Here's how the part is built. I have some questions about the finished solid (model axes, mm). Face numbers are marked on the shaded views. Round coordinates to 2 decimals unless told otherwise and drop trailing zeros. Write each loop counter-clockwise with the first axis right and the second up, starting at its lowest first coordinate (ties: lowest second). Pieces come first, ordered by that corner, then holes. Notation, with made-up numbers: (67.5, -27) -> (87.5, -27) arc R27 ccw to (87.5, 0) -> close; hole circle Ø6 at (73.25, 22). An arc over 180 degrees is marked (long way). Put each result on its own line as item: value. Start each with the question number.
1) If I drill on line 1 along Z through (x, y) = (-20, 6.5); line 2 along Z through (x, y) = (34, -0.5); line 3 along X through (y, z) = (5, -7.25), over which ranges is the centre line in solid material (lowest first)? Write a range as [from, to].
2) I want a section at C-C, the plane z = -9. List the corners of the cut face in (x, y) for me, then the cut area to 3 significant figures.
3) I want a section at A-A, the plane x = -5. List the corners of the cut face in (y, z) for me.
4) I want a section at B-B, the plane y = 5. List the corners of the cut face in (x, z) for me, then the cut area to 3 significant figures.
5) Will these pins go through, and if not, where does the flat tip stop? P1, Ø0.6, axis at y = 9, z = 1.5, coming from the +X side; P2, Ø8, axis at x = -8, z = -2, coming from the +Y side; P3, Ø4, axis at x = 14.5, y = 5, coming from the +Z side; P4, Ø1.6, axis at x = -33, z = 1.5, coming from the -Y side.
6) We'd pull the mould along Z, two halves only. Please class the marked faces 1 and 2: released by +Z, released by -Z, zero draft, split by the parting line, or undercut.
from build123d import *

# Parameters (mm, degrees)
SKIZZE1_W                            = 155
SKIZZE1_H                            = 23
SKIZZE1_W_2                          = 147
SKIZZE1_H_2                          = 15
AUFSATZ_LINEAR_AUSTRAGEN1_DEPTH      = 10
SKIZZE2_W                            = 2
SKIZZE2_H                            = 15
AUFSATZ_LINEAR_AUSTRAGEN2_DEPTH      = 2
AUFSATZ_LINEAR_AUSTRAGEN3_DEPTH      = 1.5
AUFSATZ_LINEAR_AUSTRAGEN3_DEPTH_BACK = 2
SKIZZE3_W                            = 159
SKIZZE3_H                            = 27
SKIZZE3_W_2                          = 155
SKIZZE3_H_2                          = 23


with BuildPart() as part:
    # Skizze1 → Aufsatz-Linear austragen1 (new body)
    with BuildSketch(Plane(origin=(0, 0, 0), x_dir=(1, 0, 0), z_dir=(0, 1, 0))):
        Rectangle(SKIZZE1_W, SKIZZE1_H)
        Rectangle(SKIZZE1_W_2, SKIZZE1_H_2, mode=Mode.SUBTRACT)
    extrude(amount=AUFSATZ_LINEAR_AUSTRAGEN1_DEPTH)

    # Skizze2 → Aufsatz-Linear austragen2 (add)
    with BuildSketch(Plane(origin=(0, 10, 0), x_dir=(1, 0, 0), z_dir=(0, 1, 0))):
        with Locations((-52.5, 0)):
            Rectangle(SKIZZE2_W, SKIZZE2_H)
        with Locations((-32.5, 0)):
            Rectangle(SKIZZE2_W, SKIZZE2_H)
        with Locations((-12.5, 0)):
            Rectangle(SKIZZE2_W, SKIZZE2_H)
        with Locations((7.5, 0)):
            Rectangle(SKIZZE2_W, SKIZZE2_H)
        with Locations((27.5, 0)):
            Rectangle(SKIZZE2_W, SKIZZE2_H)
        with Locations((47.5, 0)):
            Rectangle(SKIZZE2_W, SKIZZE2_H)
    extrude(amount=-AUFSATZ_LINEAR_AUSTRAGEN2_DEPTH)

    # Skizze3 → Aufsatz-Linear austragen3 (add, two sides: drawn at the far end of the back side and taken through both)
    with BuildSketch(Plane.XZ.offset(-AUFSATZ_LINEAR_AUSTRAGEN3_DEPTH_BACK)):
        Rectangle(SKIZZE3_W, SKIZZE3_H)
        Rectangle(SKIZZE3_W_2, SKIZZE3_H_2, mode=Mode.SUBTRACT)
    extrude(amount=AUFSATZ_LINEAR_AUSTRAGEN3_DEPTH + AUFSATZ_LINEAR_AUSTRAGEN3_DEPTH_BACK)


solid = part.part
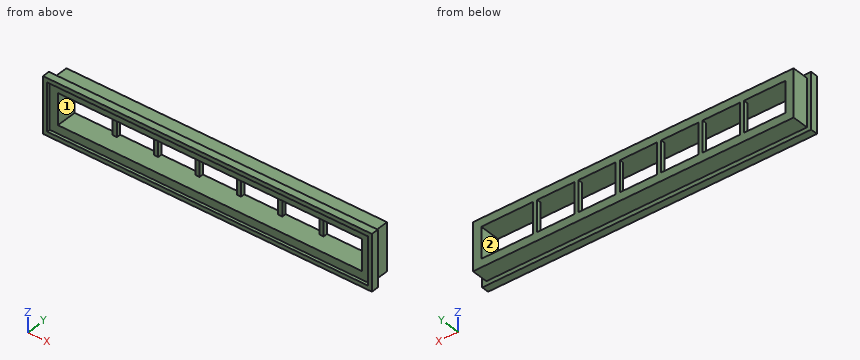
Findings:
1. line 1: z = [-11.5, -7.5], [7.5, 11.5]
1. line 2: z = [-13.5, -11.5], [11.5, 13.5]
1. line 3: x = [-77.5, -73.5], [73.5, 77.5]
2. outline: (-79.5, -1.5) -> (-77.5, -1.5) -> (-77.5, 0) -> (77.5, 0) -> (77.5, -1.5) -> (79.5, -1.5) -> (79.5, 2) -> (77.5, 2) -> (77.5, 10) -> (-77.5, 10) -> (-77.5, 2) -> (-79.5, 2) -> close
2. area: 1,560 mm2
3. outline: (-1.5, -13.5) -> (2, -13.5) -> (2, -11.5) -> (10, -11.5) -> (10, -7.5) -> (0, -7.5) -> (0, -11.5) -> (-1.5, -11.5) -> close; (-1.5, 11.5) -> (0, 11.5) -> (0, 7.5) -> (10, 7.5) -> (10, 11.5) -> (2, 11.5) -> (2, 13.5) -> (-1.5, 13.5) -> close
4. outline: (-77.5, -11.5) -> (77.5, -11.5) -> (77.5, 11.5) -> (-77.5, 11.5) -> close; hole (-73.5, -7.5) -> (73.5, -7.5) -> (73.5, 7.5) -> (-73.5, 7.5) -> close
4. area: 1,360 mm2
5. P1: stops at x = 77.5
5. P2: stops at y = 10
5. P3: stops at z = 11.5
5. P4: stops at y = 8
6. face 1: undercut
6. face 2: undercut
